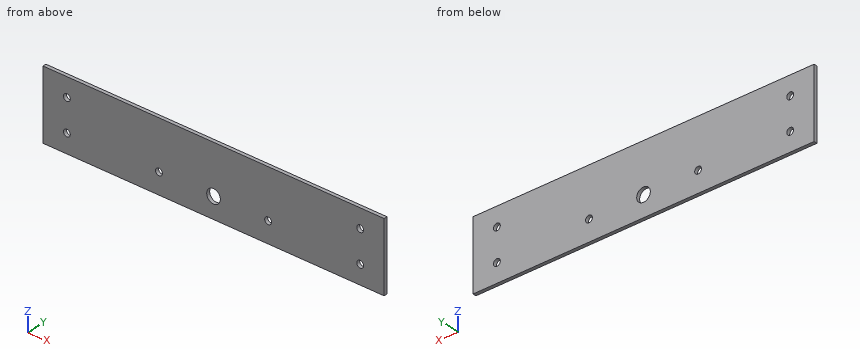
from build123d import *

# Parameters (mm, degrees)
SKETCH1_W           = 500
SKETCH1_H           = 100
BOSS_EXTRUDE1_DEPTH = 5
SKETCH3_R           = 10
CUT_EXTRUDE1_DEPTH  = 510.926465287
SKETCH4_R           = 5
CUT_EXTRUDE2_DEPTH  = 510.926465287
SKETCH5_R           = 5
CUT_EXTRUDE3_DEPTH  = 510.926465287
SKETCH7_R           = 5
CUT_EXTRUDE4_DEPTH  = 510.926465287


with BuildPart() as part:
    # Sketch1 → Boss-Extrude1 (new body)
    with BuildSketch(Plane(origin=(0, 0, 0), x_dir=(1, 0, 0), z_dir=(0, 1, 0))):
        with Locations((250, 50)):
            Rectangle(SKETCH1_W, SKETCH1_H)
    extrude(amount=BOSS_EXTRUDE1_DEPTH)

    # Sketch3 → Cut-Extrude1 (cut, through all)
    with BuildSketch(Plane(origin=(0, 5, 0), x_dir=(1, 0, 0), z_dir=(0, 1, 0))):
        with Locations(Location((250, 70, 0), (0, 0, 270))):
            Circle(SKETCH3_R)
    extrude(amount=-CUT_EXTRUDE1_DEPTH, mode=Mode.SUBTRACT)

    # Sketch4 → Cut-Extrude2 (cut, through all)
    with BuildSketch(Plane(origin=(0, 5, 0), x_dir=(1, 0, 0), z_dir=(0, 1, 0))):
        with Locations(Location((170, 70, 0), (0, 0, 270))):
            Circle(SKETCH4_R)
    extrude(amount=-CUT_EXTRUDE2_DEPTH, mode=Mode.SUBTRACT)

    # Sketch5 → Cut-Extrude3 (cut, through all)
    with BuildSketch(Plane(origin=(0, 5, 0), x_dir=(1, 0, 0), z_dir=(0, 1, 0))):
        with Locations(Location((330, 70, 0), (0, 0, 270))):
            Circle(SKETCH5_R)
    extrude(amount=-CUT_EXTRUDE3_DEPTH, mode=Mode.SUBTRACT)

    # Sketch7 → Cut-Extrude4 (cut, through all)
    with BuildSketch(Plane(origin=(0, 0, 0), x_dir=(-1, 0, 0), z_dir=(0, -1, 0))):
        with Locations(Location((-465, 73, 0), (0, 0, 90))):
            Circle(SKETCH7_R)
        with Locations(Location((-465, 27, 0), (0, 0, 90))):
            Circle(SKETCH7_R)
        with Locations(Location((-35, 27, 0), (0, 0, 90))):
            Circle(SKETCH7_R)
        with Locations(Location((-35, 73, 0), (0, 0, 90))):
            Circle(SKETCH7_R)
    extrude(amount=-CUT_EXTRUDE4_DEPTH, mode=Mode.SUBTRACT)


solid = part.part
Read the model definition and answer for the solid it produces. Units are mm, in the model's axes. Coordinates: 2 decimals unless noted, no trailing zeros. Loops run counter-clockwise (first coordinate to the right, second up) from the corner with the lowest first, then second, coordinate; pieces in that order, holes last.
Q1. Consider probe 1 along X at (y, z) = (3.1, -27); probe 2 along X at (y, z) = (2.6, -28); probe 3 along X at (y, z) = (1.95, -63.5). Determine where each line is inside the solid, lowest interval first.
Q2. The part is cut by section D-D on x = 250. Write down the section's boundary in (y, z).
Q3. The part is cut by section C-C on y = 1.5. Write down the section's boundary in (x, z), and give its area (3 significant figures).
Q4. The part is cut by section A-A on x = 465. Write down the section's boundary in (y, z).
Q5. The part is cut by section B-B on x = 170. Write down the section's boundary in (y, z).
Results below:
1. probe 1: x = 0 to 30, 40 to 460, 470 to 500
1. probe 2: x = 0 to 30.1, 39.9 to 460.1, 469.9 to 500
1. probe 3: x = 0 to 242.4, 257.6 to 500
2. outline: (0, -100) - (5, -100) - (5, -80) - (0, -80) - close; (0, -60) - (5, -60) - (5, 0) - (0, 0) - close
3. outline: (0, -100) - (500, -100) - (500, 0) - (0, 0) - close; hole circle Ø10 at (35, -73); hole circle Ø10 at (35, -27); hole circle Ø10 at (170, -70); hole circle Ø20 at (250, -70); hole circle Ø10 at (330, -70); hole circle Ø10 at (465, -73); hole circle Ø10 at (465, -27)
3. area: 49,200 mm2
4. outline: (0, -100) - (5, -100) - (5, -78) - (0, -78) - close; (0, -68) - (5, -68) - (5, -32) - (0, -32) - close; (0, -22) - (5, -22) - (5, 0) - (0, 0) - close
5. outline: (0, -100) - (5, -100) - (5, -75) - (0, -75) - close; (0, -65) - (5, -65) - (5, 0) - (0, 0) - close
